from build123d import *

# Parameters (mm, degrees)
FILLET1_R     = 0.25
CHAMFER1_SIZE = 0.5


with BuildPart() as part:
    # Sketch1 → Revolve1 (revolve)
    with BuildSketch(Plane.XY, mode=Mode.PRIVATE) as revolve1_sk:
        with BuildLine():
            Line((0, 5), (0, 1.85))
            Line((0, 1.85), (4, 1.85))
            Line((4, 1.85), (4, 5))
            Line((4, 5), (3, 5))
            Line((3, 5), (3, 4))
            ThreePointArc((3, 4), (2, 3), (1, 4))
            Line((1, 4), (1, 5))
            Line((1, 5), (0, 5))
        make_face()
    revolve(revolve1_sk.sketch.rotate(Axis((0, 0, 0), (1, 0, 0)), 90), axis=Axis((0, 0, 0), (1, 0, 0)))

    # Fillet1
    fillet1_edges = [part.edges().sort_by_distance(p)[0] for p in [
        (1, 0, -5),
        (3, 0, -5),
    ]]
    fillet(fillet1_edges, radius=FILLET1_R)

    # Chamfer1
    chamfer1_edges = [part.edges().sort_by_distance(p)[0] for p in [
        (0, 0, -5),
        (4, 0, -5),
        (4, 0, -1.85),
        (0, 0, -1.85),
    ]]
    chamfer(chamfer1_edges, length=CHAMFER1_SIZE)


solid = part.part
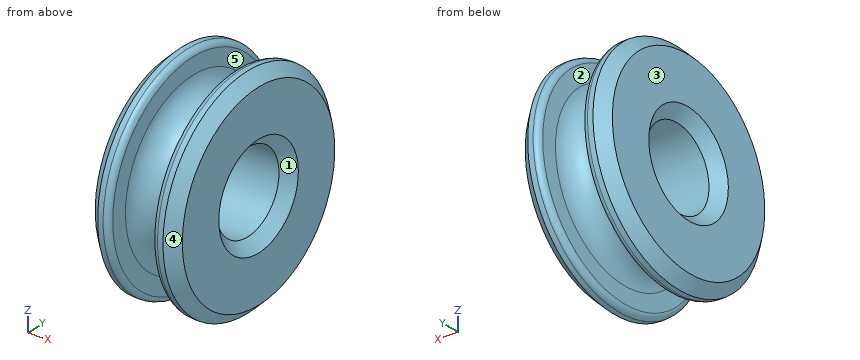
Check sheet for the modelled part. Datum: model origin and axes. Units: mm. Face numbers are marked on the shaded views. A direction names the side the tool comes from. Round coordinates to 2 decimals unless told otherwise and drop trailing zeros. Order: outer loops, then holes, each group sorted by start corner. A loop starts at its lowest first (then second) coordinate and runs counter-clockwise, first axis right, second up. Notation, with made-up numbers: M 15,-36.75 L 28,-36.75 A24 ccw 28,1.25 Z; hole C 62,49.5 d10. An arc over 180 degrees is marked long. One line per item, written item: value. Start each with the question number.
1. Scan lines: line 1 along X through (y, z) = (-2, 3.75); line 2 along Y through (x, z) = (2.45, 0); line 3 along Y through (x, z) = (1.4, 0). Record each from-to range of solid material in increasing order.
2. Release check for a two-part mould opening along X. For the marked faces 3, 4 and 5 record: released by +X, released by -X, zero draft, split by the parting line, or undercut.
3. Section check C-C on x = 0.35. Enter the section's corners in (y, z), and give its area (3 significant figures).
4. Gauge pin test, flat ends, axial feed: P1, Ø1, axis at x = 3, z = 1.5, coming from the +Y side; P2, Ø1.5, axis at x = 2.5, z = -2, coming from the +Y side; P3, Ø1.5, axis at x = 3.5, y = -2.5, coming from the +Z side; P4, Ø2, axis at y = 0, z = 0, coming from the +X side. Record the tip position at first contact, or that the pin passes through.
5. Access from +Z, -Z, +X, -X, +Y, -Y to the whole of each face (thin tool, end or side, straight path). Record for the marked faces 1 and 2.
6. Section check A-A on z = 0. Enter the section's corners in (x, y), and give its area (3 significant figures).
7. Section check D-D on x = 1.2. Enter the section's corners in (y, z), and give its area (3 significant figures).
Results found:
1. line 1: 0 to 1, 3 to 4
1. line 2: -3.11 to -1.85, 1.85 to 3.11
1. line 3: -3.2 to -1.85, 1.85 to 3.2
2. face 3: released by -X
2. face 4: released by +X
2. face 5: undercut
3. outline: C 0,0 d9.7; hole C 0,0 d4
3. area: 61.3 mm^2
4. P1: y = 4.89
4. P2: y = 4.71
4. P3: z = 4.68
4. P4: through
5. face 1: +X
5. face 2: none
6. outline: M 0,-4.5 L 0.5,-5 L 0.75,-5 A0.25 ccw 1,-4.75 L 1,-4 A1 cw 3,-4 L 3,-4.75 A0.25 ccw 3.25,-5 L 3.5,-5 L 4,-4.5 L 4,-2.35 L 3.5,-1.85 L 0.5,-1.85 L 0,-2.35 Z; M 0,2.35 L 0.5,1.85 L 3.5,1.85 L 4,2.35 L 4,4.5 L 3.5,5 L 3.25,5 A0.25 ccw 3,4.75 L 3,4 A1 cw 1,4 L 1,4.75 A0.25 ccw 0.75,5 L 0.5,5 L 0,4.5 Z
6. area: 17.0 mm^2
7. outline: C 0,0 d6.8; hole C 0,0 d3.7
7. area: 25.6 mm^2
